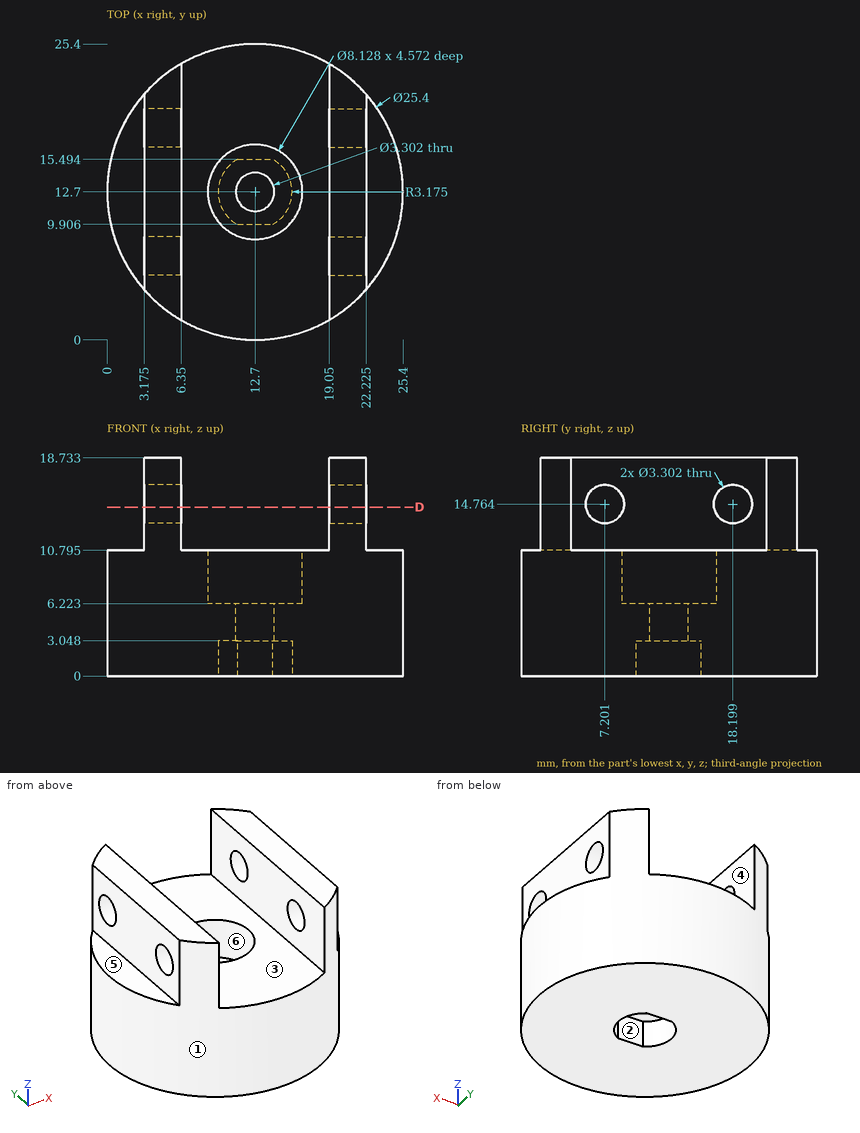
Answer from the drawing. Dimensions are ordinates in mm from the lowest x, y and z of the part. A direction names the side the tool comes from. Give positions to 0.01 mm unless a question says otherwise; leave off trailing zeros. Use a Markdown table: item, result.
Q1. A tool of negligible diameter and unlimited length cuts with its end or side. For the marked faces 4, 5 and 6, from which of +Z, -Z, +X, -X, +Y, -Y can it reach the whole face along a straight path? Write none if from no direction.
Solved:
| item | result |
|---|---|
| face 4 | +Z, +Y, -Y |
| face 5 | +Z, -X, +Y, -Y |
| face 6 | +Z |
Q2. Find the intervals of material crossed by line 1 along X through (y, z) = (12.7, 4); line 2 along Y through (x, z) = (12.7, 7.35) (1 decimal); line 3 along Z through (x, y) = (14.75, 12), in increasing order.
Solved:
| item | result |
|---|---|
| line 1 | x = 0 to 11.05, 14.35 to 25.4 |
| line 2 | y = 0 to 8.6, 16.8 to 25.4 |
| line 3 | z = 3.05 to 6.22 |
Q3. Each of these flat-tipped pins is pushed along its axis until it touches: pin 1 (10 mm diameter, centred on x = 11, y = 7.5, fed in from +Z); pin 2 (6.5 mm diameter, centred on y = 14.5, z = 16, fed in from -X) (1 decimal); pin 3 (2.5 mm diameter, centred on x = 1, y = 13.5, fed in from +Z) (1 decimal); pin 4 (10 mm diameter, centred on x = 18, z = 15.5, fed in from +Y) (1 decimal). Where does it stop, or does it pass through?
Solved:
| item | result |
|---|---|
| pin 1 | stops at z = 18.73 |
| pin 2 | stops at x = 3.2 |
| pin 3 | stops at z = 10.8 |
| pin 4 | stops at y = 24.9 |
Q4. Section D-D, the plane z = 14.5 is taken. Count the separate pieces of the cut face and the enclosed holes in it.
Solved:
| item | result |
|---|---|
| separate pieces | 6 |
| enclosed holes | 0 |
Q5. Determine the mould class of the marked faces 1, 2 and 3 for opening direction Y: pulls with the +Y half, pulls with the -Y half, needs draft (parallel to the pull), parting line crosses it, or undercut.
Solved:
| item | result |
|---|---|
| face 1 | parting line crosses it |
| face 2 | undercut |
| face 3 | needs draft |
